from build123d import *

# Parameters (mm, degrees)
SKETCH1_R           = 1.5
BOSS_EXTRUDE1_DEPTH = 2.5
BOSS_EXTRUDE2_DEPTH = 10
FILLET1_R           = 2
SKETCH3_R           = 2.5
CUT_EXTRUDE1_DEPTH  = 5
SKETCH4_R           = 5
SKETCH4_R_2         = 4.5
CUT_EXTRUDE2_DEPTH  = 0.5
SKETCH5_W           = 10
SKETCH5_H           = 6
SKETCH5_R           = 0.5
CUT_EXTRUDE3_DEPTH  = 5


with BuildPart() as part:
    # Sketch1 → Boss-Extrude1 (new body)
    with BuildSketch(Plane.XY):
        with BuildLine():
            Line((-26, 28), (26, 28))
            ThreePointArc((26, 28), (27.414213562, 27.414213562), (28, 26))
            Line((28, 26), (28, -26))
            ThreePointArc((28, -26), (27.414213562, -27.414213562), (26, -28))
            Line((26, -28), (-26, -28))
            ThreePointArc((-26, -28), (-27.414213562, -27.414213562), (-28, -26))
            Line((-28, -26), (-28, 26))
            ThreePointArc((-28, 26), (-27.414213562, 27.414213562), (-26, 28))
        make_face()
        with Locations((-25, 25)):
            Circle(SKETCH1_R, mode=Mode.SUBTRACT)
        with Locations((25, 25)):
            Circle(SKETCH1_R, mode=Mode.SUBTRACT)
        with Locations((25, -25)):
            Circle(SKETCH1_R, mode=Mode.SUBTRACT)
        with Locations((-25, -25)):
            Circle(SKETCH1_R, mode=Mode.SUBTRACT)
    extrude(amount=BOSS_EXTRUDE1_DEPTH)

    # Sketch2 → Boss-Extrude2 (add)
    with BuildSketch(Plane.XY.offset(2.5)):
        Polygon((-11.597979746, -28), (11.597979746, -28), (28, -11.597979746), (28, 11.597979746), (11.597979746, 28), (-11.597979746, 28), (-28, 11.597979746), (-28, -11.597979746), align=None)
    extrude(amount=BOSS_EXTRUDE2_DEPTH)

    # Fillet1
    fillet1_edges = [part.edges().sort_by_distance(p)[0] for p in [
        (11.597979746, -28, 7.5),
        (28, -11.597979746, 7.5),
        (28, 11.597979746, 7.5),
        (11.597979746, 28, 7.5),
        (-11.597979746, 28, 7.5),
        (-28, 11.597979746, 7.5),
        (-28, -11.597979746, 7.5),
        (-11.597979746, -28, 7.5),
    ]]
    fillet(fillet1_edges, radius=FILLET1_R)

    # Sketch3 → Cut-Extrude1 (cut)
    with BuildSketch(Plane(origin=(0, 0, 0), x_dir=(-1, 0, 0), z_dir=(0, 0, -1))):
        Circle(SKETCH3_R)
    extrude(amount=-CUT_EXTRUDE1_DEPTH, mode=Mode.SUBTRACT)

    # Sketch4 → Cut-Extrude2 (cut)
    with BuildSketch(Plane(origin=(0, 0, 0), x_dir=(-1, 0, 0), z_dir=(0, 0, -1))):
        Circle(SKETCH4_R)
        Circle(SKETCH4_R_2, mode=Mode.SUBTRACT)
    extrude(amount=-CUT_EXTRUDE2_DEPTH, mode=Mode.SUBTRACT)

    # Sketch5 → Cut-Extrude3 (cut)
    with BuildSketch(Plane.XZ.offset(28)):
        with Locations((0, 7.5)):
            Rectangle(SKETCH5_W, SKETCH5_H)
        with Locations((-3, 7.5)):
            Circle(SKETCH5_R, mode=Mode.SUBTRACT)
        with Locations((-1, 7.5)):
            Circle(SKETCH5_R, mode=Mode.SUBTRACT)
        with Locations((1, 7.5)):
            Circle(SKETCH5_R, mode=Mode.SUBTRACT)
        with Locations((3, 7.5)):
            Circle(SKETCH5_R, mode=Mode.SUBTRACT)
    extrude(amount=-CUT_EXTRUDE3_DEPTH, mode=Mode.SUBTRACT)


solid = part.part
Design review of the part built by this model. Coordinates are the model's own, in mm. A direction names the side the tool comes from. Give positions to 0.01 mm unless a question says otherwise; leave off trailing zeros. Loops run counter-clockwise (first coordinate to the right, second up) from the corner with the lowest first, then second, coordinate; pieces in that order, holes last. Notation, with made-up numbers: M 84.5,59.5 L 106.5,59.5 A26 ccw 106.5,96.5 Z; hole C 41,75 d2. An arc over 180 degrees is marked long. Answer as a JSON object with one key per item and string values.
Item 1: Wall thickness on line 1 along Y through (x, z) = (25, 1.4); line 2 along Y through (x, z) = (11, 9.75); line 3 along Y through (x, z) = (24, 11.5): over which ranges is each line inside the solid? List them lowest first.
Output values:
{"line 1": "y = -28 to -26.5, -23.5 to 23.5, 26.5 to 28", "line 2": "y = -27.99 to 27.99", "line 3": "y = -15.6 to 15.6"}
Item 2: We need section A-A (z = 1.25). State the section outline as (x, y) points.
Output values:
{"outline": "M -28,-26 A2 ccw -26,-28 L 26,-28 A2 ccw 28,-26 L 28,26 A2 ccw 26,28 L -26,28 A2 ccw -28,26 Z; hole C -25,-25 d3; hole C -25,25 d3; hole C 0,0 d5; hole C 25,-25 d3; hole C 25,25 d3"}
Item 3: For P1, Ø5, axis at x = 25, y = -25, coming from the +Z side; P2, Ø2.5, axis at x = -0.5, y = 0, coming from the -Z side; P3, Ø2.5, axis at y = -26, z = 7.5, coming from the -X side, all flat-tipped, find the tip position at first contact; note any pin that passes through.
Output values:
{"P1": "stops at z = 2.5", "P2": "stops at z = 5", "P3": "stops at x = -14.85"}
Item 4: Mouldability with a two-part tool opening along Z and no side actions: class faces 1 (the face through (0, -23, 8)), 2 (the face through (-19.7, 19.9, 7.4)), 3 (the face through (23, 23, 2.5)) as pulls with the +Z half, pulls with the -Z half, needs draft (parallel to the pull), parting line crosses it, or undercut.
Output values:
{"face 1": "undercut", "face 2": "needs draft", "face 3": "pulls with the +Z half"}
Item 5: Machinability: for faces 4 (the face through (5, -26, 7)), 5 (the face through (23, -23, 2.5)), 6 (the face through (19.9, 19.7, 7.4)), 7 (the face through (-27.852, 11.525, 7.57)), which of the approach directions +Z, -Z, +X, -X, +Y, -Y give a long, thin tool a straight path to every point of the face, cutting with its end or side? Answer none if there is none.
Output values:
{"face 4": "-Y", "face 5": "+Z, +X, -Y", "face 6": "+Z, +X, +Y", "face 7": "+Z, -X, +Y"}
Item 6: We need section B-B (y = -18). State the section outline as (x, z) points.
Output values:
{"outline": "M -28,0 L 28,0 L 28,2.5 L 21.6,2.5 L 21.6,12.5 L -21.6,12.5 L -21.6,2.5 L -28,2.5 Z"}
Item 7: We need section D-D (y = -1). State the section outline as (x, z) points, and give its area (3 significant figures).
Output values:
{"outline": "M -28,0 L -4.9,0 L -4.9,0.5 L -4.39,0.5 L -4.39,0 L -2.29,0 L -2.29,5 L 2.29,5 L 2.29,0 L 4.39,0 L 4.39,0.5 L 4.9,0.5 L 4.9,0 L 28,0 L 28,12.5 L -28,12.5 Z", "area": "677 mm2"}
Item 8: We need section C-C (x = -21). State the section outline as (y, z) points.
Output values:
{"outline": "M -28,0 L 28,0 L 28,2.5 L 18.6,2.5 L 18.6,12.5 L -18.6,12.5 L -18.6,2.5 L -28,2.5 Z"}
